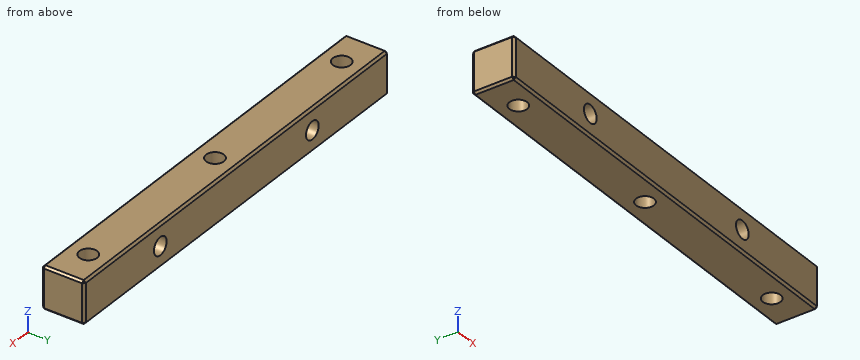
```python
from build123d import *

# Parameters (mm, degrees)
SKETCH_1_W         = 60
SKETCH_1_H         = 6
EXTRUDE_1_DEPTH    = 3
HOLE_WIZARD_M3_1_D = 2.5
HOLE_WIZARD_M3_2_D = 2.5
CHAMFER_1_SIZE     = 0.3


with BuildPart() as part:
    # 草图1 → 凸台-拉伸1 (new, symmetric)
    with BuildSketch(Plane.XY):
        Rectangle(SKETCH_1_W, SKETCH_1_H)
    extrude(amount=EXTRUDE_1_DEPTH, both=True)

    # M3 螺纹孔1 (through all)
    with Locations(Plane.XY.offset(3)):
        with Locations((-25, 0), (0, 0), (25, 0)):
            Hole(HOLE_WIZARD_M3_1_D / 2)

    # M3 螺纹孔2 (through all)
    with Locations(Plane(origin=(0, 3, 0), x_dir=(1, 0, 0), z_dir=(0, 1, 0))):
        with Locations((-15, 0), (15, 0)):
            Hole(HOLE_WIZARD_M3_2_D / 2)

    # 倒角1
    chamfer_1_edges = [part.edges().sort_by_distance(p)[0] for p in [
        (-30, 0, 3),
        (0, -3, 3),
        (30, 0, 3),
        (0, -3, -3),
        (-30, 0, -3),
        (0, 3, -3),
        (30, 0, -3),
        (30, -3, 0),
        (-30, -3, 0),
        (-30, 3, 0),
        (30, 3, 0),
        (0, 3, 3),
    ]]
    chamfer(chamfer_1_edges, length=CHAMFER_1_SIZE)


solid = part.part
```
Could you check a few things on this model? Use its own coordinates, in mm. Coordinates: 2 decimals unless noted, no trailing zeros. Loops run counter-clockwise (first coordinate to the right, second up) from the corner with the lowest first, then second, coordinate; pieces in that order, holes last. Notation, with made-up numbers: M 52.5,33.25 L 77.5,33.25 A37 cw 77.5,72.25 Z; hole C 64,29.5 d10. An arc over 180 degrees is marked long. Put each result on its own line as item: value. Start each with the question number.
(1) Suppose I cut it at A-A on y = 0. Please give me the cut outline in (x, z), then the cut area to 3 significant figures.
(2) Suppose I cut it at B-B on z = 0. Please give me the cut outline in (x, y), then the cut area to 3 significant figures.
(3) Suppose I cut it at C-C on x = -25. Please give me the cut outline in (y, z).
(4) I need wall thicknesses on line 1 (Y direction, x = 25, z = 0.75); line 2 (X direction, y = -1.75, z = 1). Which ranges of each line are inside material? Lowest first, please. Write a range as from..to.
(5) Will these pins go through, and if not, where does the flat tip stop? P1, Ø3, axis at x = 15, z = 0, coming from the -Y side; P2, Ø2, axis at x = -25, y = 0, coming from the +Z side.
Solutions:
1. outline: M -30,-2.7 L -29.7,-3 L -26.25,-3 L -26.25,3 L -29.7,3 L -30,2.7 Z; M -23.75,-3 L -1.25,-3 L -1.25,3 L -23.75,3 Z; M 1.25,-3 L 23.75,-3 L 23.75,3 L 1.25,3 Z; M 26.25,-3 L 29.7,-3 L 30,-2.7 L 30,2.7 L 29.7,3 L 26.25,3 Z; hole C -15,0 d2.5; hole C 15,0 d2.5
1. area: 305 mm2
2. outline: M -30,-2.7 L -29.7,-3 L -16.25,-3 L -16.25,3 L -29.7,3 L -30,2.7 Z; M -13.75,-3 L 13.75,-3 L 13.75,3 L -13.75,3 Z; M 16.25,-3 L 29.7,-3 L 30,-2.7 L 30,2.7 L 29.7,3 L 16.25,3 Z; hole C -25,0 d2.5; hole C 0,0 d2.5; hole C 25,0 d2.5
2. area: 315 mm2
3. outline: M -3,-2.7 L -2.7,-3 L -1.25,-3 L -1.25,3 L -2.7,3 L -3,2.7 Z; M 1.25,-3 L 2.7,-3 L 3,-2.7 L 3,2.7 L 2.7,3 L 1.25,3 Z
4. line 1: y = -3..-1.25, 1.25..3
4. line 2: x = -30..-15.75, -14.25..14.25, 15.75..30
5. P1: stops at y = -3
5. P2: passes through
